from build123d import *

# Parameters (mm, degrees)
SKETCH_1_R      = 1.6
EXTRUDE_1_DEPTH = 1


with BuildPart() as part:
    # 草图1 → 凸台-拉伸1 (new body)
    with BuildSketch(Plane.XY):
        Polygon((26, 0), (-26, 0), (-26, 17), (-5, 35), (5, 35), (26, 17), align=None)
        with Locations((-13.725, 19)):
            Circle(SKETCH_1_R, mode=Mode.SUBTRACT)
        with Locations(Location((13.725, 19, 0), (0, 0, 180))):
            Circle(SKETCH_1_R, mode=Mode.SUBTRACT)
        with Locations((-23, 4)):
            Circle(SKETCH_1_R, mode=Mode.SUBTRACT)
        with Locations(Location((20, 4, 0), (0, 0, 180))):
            Circle(SKETCH_1_R, mode=Mode.SUBTRACT)
        with Locations((0, 31.5)):
            Circle(SKETCH_1_R, mode=Mode.SUBTRACT)
    extrude(amount=EXTRUDE_1_DEPTH)


solid = part.part
Design review of the part built by this model. Coordinates are the model's own, in mm. Round coordinates to 2 decimals unless told otherwise and drop trailing zeros. Write each loop counter-clockwise with the first axis right and the second up, starting at its lowest first coordinate (ties: lowest second). Pieces come first, ordered by that corner, then holes. Notation, with made-up numbers: M -17.75,41 L 27.25,41 A22 ccw 27.25,57 Z; hole C -3,39 d4. An arc over 180 degrees is marked long. One line per item, written item: value. Start each with the question number.
1. Draft analysis for pull direction X (two halves, no side actions). For faces 1 (the face through (-21.474, 4.481, 0.493)), 2 (the face through (15.35, 26.13, 0.49)), 3 (the face through (0, 14, 1)), state which applies: pulls with the +X half, pulls with the -X half, needs draft (parallel to the pull), parting line crosses it, or undercut.
2. To check wall thickness, follow probe 1 along Y at (x, z) = (0, 0.6); probe 2 along X at (y, z) = (19.5, 0.5); probe 3 along Y at (x, z) = (19.5, 0.7). State the ranges of each line that lie inside material, in increasing order. Write a range as from..to.
3. Take a section at D-D on y = 31.5. State the section outline as (x, z) points.
4. Clearance check with a flat-ended pin moving along its axis: P1, Ø2.5, axis at x = 20, y = 4, coming from the +Z side. State where the tip first meets the part, or that it passes through.
5. Take a section at B-B on y = 4. State the section outline as (x, z) points, then the cut area to 3 significant figures.
6. Take a section at A-A on x = 0. State the section outline as (y, z) points.
7. Take a section at C-C on z = 0.15. State the section outline as (x, y) points (3 decimals), then the cut area to 3 significant figures.
Computed:
1. face 1: undercut
1. face 2: pulls with the +X half
1. face 3: needs draft
2. probe 1: y = 0..29.9, 33.1..35
2. probe 2: x = -23.08..-15.24, -12.21..12.21, 15.24..23.08
2. probe 3: y = 0..2.48, 5.52..22.57
3. outline: M -9.08,0 L -1.6,0 L -1.6,1 L -9.08,1 Z; M 1.6,0 L 9.08,0 L 9.08,1 L 1.6,1 Z
4. P1: passes through
5. outline: M -26,0 L -24.6,0 L -24.6,1 L -26,1 Z; M -21.4,0 L 18.4,0 L 18.4,1 L -21.4,1 Z; M 21.6,0 L 26,0 L 26,1 L 21.6,1 Z
5. area: 45.6 mm²
6. outline: M 0,0 L 29.9,0 L 29.9,1 L 0,1 Z; M 33.1,0 L 35,0 L 35,1 L 33.1,1 Z
7. outline: M -26,0 L 26,0 L 26,17 L 5,35 L -5,35 L -26,17 Z; hole C -23,4 d3.2; hole C -13.725,19 d3.2; hole C 0,31.5 d3.2; hole C 13.725,19 d3.2; hole C 20,4 d3.2
7. area: 1,400 mm²
